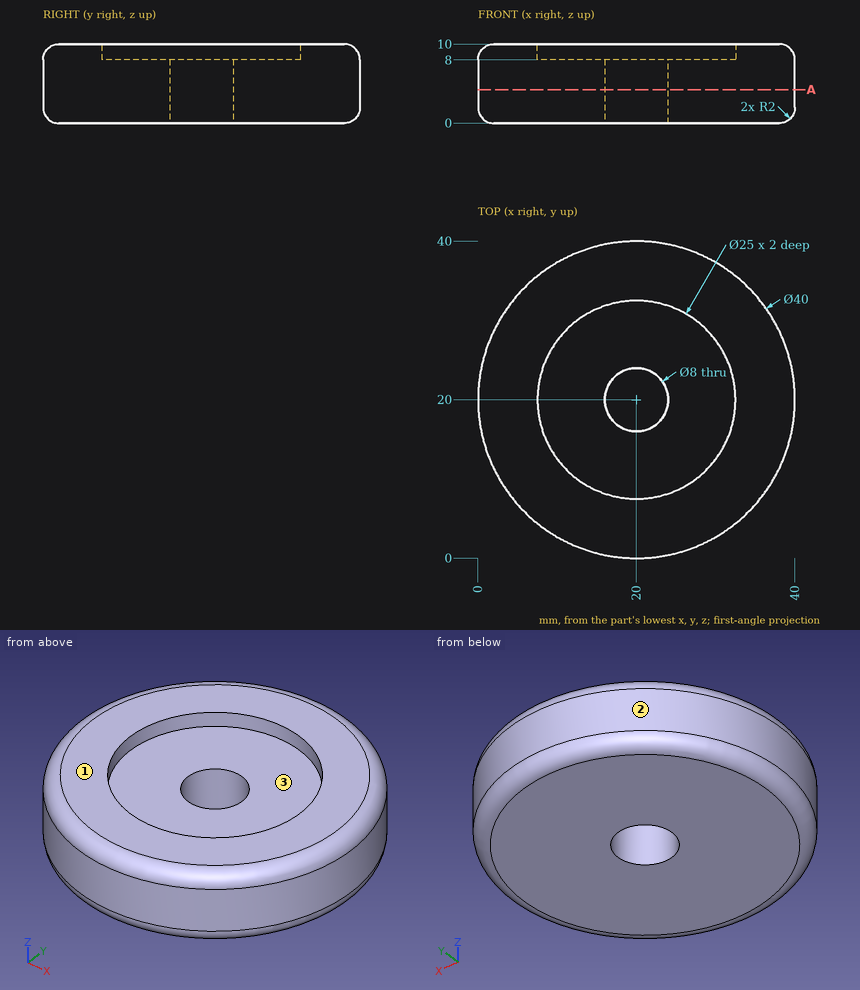
Source: three-view drawing plus pictorial views. Frame: mm from the lowest corner of the part. Give positions to 0.01 mm unless a question says otherwise; leave off trailing zeros. Loops run counter-clockwise (first coordinate to the right, second up) from the corner with the lowest first, then second, coordinate; pieces in that order, holes last.
1) Contact query for flat-ended pins moving along their axis: pin 1 (1.5 mm diameter, centred on x = 18.5, z = 4.5, fed in from +Y); pin 2 (22.5 mm diameter, centred on x = 20, y = 20, fed in from +Z); pin 3 (1.5 mm diameter, centred on x = 18, z = 7.5, fed in from -Y). Output: stop coordinate, or through.
A:
pin 1: stops at y = 39.99
pin 2: stops at z = 8
pin 3: stops at y = 0.04
2) Line query: L1, parallel to Y at x = 20, z = 4; L2, parallel to Z at x = 11.5, y = 28.5; L3, parallel to Y at x = 9, z = 8.25. Output: solid intervals per line, ascending.
A:
L1: y = 0 to 16, 24 to 40
L2: z = 0 to 8
L3: y = 3.32 to 14.06, 25.94 to 36.68
3) Mould query, pull axis X, two halves, no side actions, for the marked faces 1, 2 and 3. Classes: released by +X, released by -X, zero draft, split by the parting line, or undercut.
A:
face 1: zero draft
face 2: split by the parting line
face 3: undercut
4) Section query A-A on z = 4.25. Return the cut outline in (x, y), and give its area (3 significant figures).
A:
outline: circle Ø40 at (20, 20); hole circle Ø8 at (20, 20)
area: 1,210 mm2
